Could you check a few things on this model? Use its own coordinates, in mm. Face numbers are marked on the shaded views. A direction names the side the tool comes from. Coordinates: 2 decimals unless noted, no trailing zeros. Loops run counter-clockwise (first coordinate to the right, second up) from the corner with the lowest first, then second, coordinate; pieces in that order, holes last.
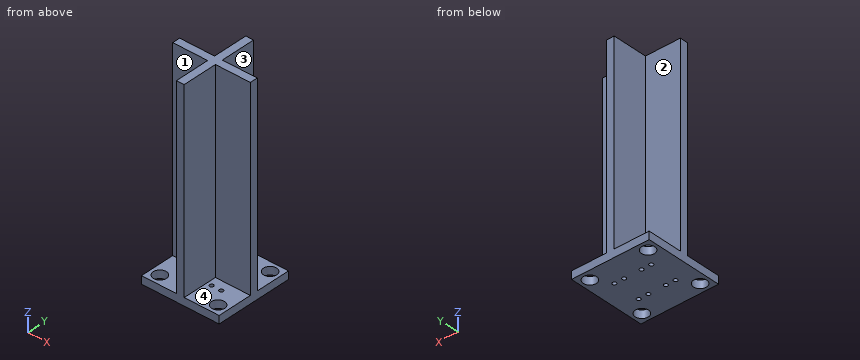
from build123d import *

# Parameters (mm, degrees)
F1_DEPTH = 1
F3_D     = 1
F4_W     = 2
F4_H     = 9
F4_H_2   = 2
F4_W_2   = 9
F5_DEPTH = 50
F6_D     = 3.4


# Not quite as in the source:
# - a feature names something its author has since deleted; it is built from what else it names


with BuildPart() as f1:
    # F0 (on Top) → F1 (new body, symmetric)
    with BuildSketch(Plane.XY):
        Polygon((10, 1), (10, 10), (1, 10), (-1, 10), (-10, 10), (-10, 1), (-10, -1), (-10, -10), (-1, -10), (1, -10), (10, -10), (10, -1), align=None)
    extrude(amount=F1_DEPTH, both=True)

    # F3 (through all)
    with Locations(Plane.XY.offset(1)):
        with Locations((-4.75, 3.5), (-2.25, 3.5), (-4.75, -3.5), (-2.25, -3.5), (2.25, 3.5), (4.75, 3.5), (4.75, -3.5), (2.25, -3.5)):
            Hole(F3_D / 2)

    # F4 (on face) → F5 (join)
    with BuildSketch(Plane.XY.offset(1)):
        with Locations((0, 5.5)):
            Rectangle(F4_W, F4_H)
        Rectangle(F4_W, F4_H_2)
        with Locations((-5.5, 0)):
            Rectangle(F4_W_2, F4_H_2)
        with Locations((5.5, 0)):
            Rectangle(F4_W_2, F4_H_2)
        with Locations((0, -5.5)):
            Rectangle(F4_W, F4_H)
    extrude(amount=F5_DEPTH)

    # F6 (through all)
    with Locations(Plane.XY.offset(1)):
        with Locations((-7.5, 7.5), (7.5, 7.5), (7.5, -7.5), (-7.5, -7.5)):
            Hole(F6_D / 2)


solid = f1.part
1) Imagine slicing it at B-B on y = 3.5. List the corners of the cut face in (x, z) for me.
2) Will these pins go through, and if not, where does the flat tip stop? pin 1 (2.5 mm diameter, centred on x = -7.5, y = -7.5, fed in from -Z); pin 2 (7 mm diameter, centred on y = -7.5, z = 37.5, fed in from +X); pin 3 (5 mm diameter, centred on x = 4, z = 29, fed in from +Y); pin 4 (5.5 mm diameter, centred on x = 7.5, y = -7.5, fed in from +Z).
3) Imagine slicing it at A-A on x = 4.75. List the corners of the cut face in (y, z) for me, plus the area to 3 significant figures.
4) Imagine slicing it at D-D on y = -7.5. List the corners of the cut face in (x, z) for me, plus the area to 3 significant figures.
5) Imagine slicing it at C-C on z = 31.5. List the corners of the cut face in (x, y) for me, plus the area to 3 significant figures.
6) If I drill on L1, parallel to Y at x = 2.25, z = -0.1; L2, parallel to Y at x = -7.5, z = -0.35; L3, parallel to X at y = 4.25, z = 43, over which ranges is the centre line in solid material (lowest first)?
7) For the marked faces 1, 2, 3 and 4, which set-ups out of +Z, -Z, +X, -X, +Y, -Y let a thin tool reach every point of the face, with its end or its side?
Solved:
1. outline: (-10, -1) - (-5.25, -1) - (-5.25, 1) - (-10, 1) - close; (-4.25, -1) - (-2.75, -1) - (-2.75, 1) - (-4.25, 1) - close; (-1.75, -1) - (1.75, -1) - (1.75, 1) - (1, 1) - (1, 51) - (-1, 51) - (-1, 1) - (-1.75, 1) - close; (2.75, -1) - (4.25, -1) - (4.25, 1) - (2.75, 1) - close; (5.25, -1) - (10, -1) - (10, 1) - (5.25, 1) - close
2. pin 1: passes through
2. pin 2: stops at x = 1
2. pin 3: stops at y = 1
2. pin 4: stops at z = 1
3. outline: (-10, -1) - (-4, -1) - (-4, 1) - (-10, 1) - close; (-3, -1) - (3, -1) - (3, 1) - (1, 1) - (1, 51) - (-1, 51) - (-1, 1) - (-3, 1) - close; (4, -1) - (10, -1) - (10, 1) - (4, 1) - close
3. area: 136 mm2
4. outline: (-10, -1) - (-9.2, -1) - (-9.2, 1) - (-10, 1) - close; (-5.8, -1) - (5.8, -1) - (5.8, 1) - (1, 1) - (1, 51) - (-1, 51) - (-1, 1) - (-5.8, 1) - close; (9.2, -1) - (10, -1) - (10, 1) - (9.2, 1) - close
4. area: 126 mm2
5. outline: (-10, -1) - (-1, -1) - (-1, -10) - (1, -10) - (1, -1) - (10, -1) - (10, 1) - (1, 1) - (1, 10) - (-1, 10) - (-1, 1) - (-10, 1) - close
5. area: 76.0 mm2
6. L1: y = -10 to -4, -3 to 3, 4 to 10
6. L2: y = -10 to -9.2, -5.8 to 5.8, 9.2 to 10
6. L3: x = -1 to 1
7. face 1: +Z, -X, -Y
7. face 2: +Z, -X, +Y
7. face 3: +Z, +X, +Y
7. face 4: +Z, +X, -Y
